Geometry check sheet. Reference: the model listing, model coordinates, mm. Face numbers are marked on the shaded views. A direction names the side the tool comes from. Give positions to 0.01 mm unless a question says otherwise; leave off trailing zeros. Loops run counter-clockwise (first coordinate to the right, second up) from the corner with the lowest first, then second, coordinate; pieces in that order, holes last.
```python
from build123d import *

# Parameters (mm, degrees)
BOSS_EXTRUDE1_DEPTH      = 50
BOSS_EXTRUDE1_DEPTH_BACK = 50
SKETCH2_R                = 50
CUT_EXTRUDE2_DEPTH       = 15
BOSS_EXTRUDE2_DEPTH      = 25
BOSS_EXTRUDE2_DEPTH_BACK = 25
SKETCH5_W                = 104.607091917
SKETCH5_H                = 30
CUT_EXTRUDE3_DEPTH       = 25
SKETCH6_W                = 40
SKETCH6_H                = 15
CUT_EXTRUDE4_DEPTH       = 81
SKETCH7_R                = 10
CUT_EXTRUDE5_DEPTH       = 61


with BuildPart() as part:
    # Sketch1 → Boss-Extrude1 (new body, two sides)
    with BuildSketch(Plane.XY) as boss_extrude1_sk:
        Polygon((0, 0), (0, 80), (30, 80), (150, 20), (150, 0), align=None)
    extrude(amount=BOSS_EXTRUDE1_DEPTH)
    extrude(boss_extrude1_sk.sketch, amount=-BOSS_EXTRUDE1_DEPTH_BACK)

    # Sketch2 → Cut-Extrude2 (cut)
    with BuildSketch(Plane.XY.offset(50)):
        Circle(SKETCH2_R)
    extrude(amount=-CUT_EXTRUDE2_DEPTH, mode=Mode.SUBTRACT)

    # Sketch4 → Boss-Extrude2 (add, two sides)
    with BuildSketch(Plane.XY) as boss_extrude2_sk:
        Polygon((70, 60), (130, 60), (130, 30), align=None)
    extrude(amount=BOSS_EXTRUDE2_DEPTH)
    extrude(boss_extrude2_sk.sketch, amount=-BOSS_EXTRUDE2_DEPTH_BACK)

    # Sketch5 → Cut-Extrude3 (cut)
    with BuildSketch(Plane(origin=(0, 60, 0), x_dir=(1, 0, 0), z_dir=(0, 1, 0))):
        with Locations((29.093290598, 0)):
            Rectangle(SKETCH5_W, SKETCH5_H)
    extrude(amount=CUT_EXTRUDE3_DEPTH, mode=Mode.SUBTRACT)

    # Sketch6 → Cut-Extrude4 (cut, through all)
    with BuildSketch(Plane.XZ):
        with Locations((100, 42.5)):
            Rectangle(SKETCH6_W, SKETCH6_H)
    extrude(amount=-CUT_EXTRUDE4_DEPTH, mode=Mode.SUBTRACT)

    # Sketch7 → Cut-Extrude5 (cut, through all)
    with BuildSketch(Plane(origin=(0, 60, 0), x_dir=(1, 0, 0), z_dir=(0, 1, 0))):
        with Locations((100, 0)):
            Circle(SKETCH7_R)
    extrude(amount=-CUT_EXTRUDE5_DEPTH, mode=Mode.SUBTRACT)


solid = part.part
```
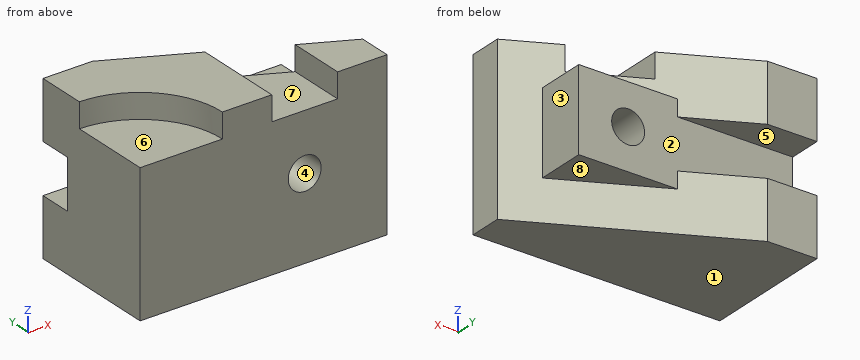
1) Sectioned sample at A-A on y = 67.5. Enter the section's corners in (x, z), plus the area to 3 significant figures.
2) Mould release check, pull along Z, two halves, no side actions. Record for the marked faces 1, 2, 3 and 4: +Z half, -Z half, draft (parallel to the pull), parting line (faces both ways), or undercut.
3) Sectioned sample at B-B on x = 100. Enter the section's corners in (y, z), plus the area to 4 significant figures.
4) Scan lines: line 1 along Z through (x, y) = (100, 43.5); line 2 along X through (y, z) = (41, 0); line 3 along X through (y, z) = (65, -30.5). Record each from-to range of solid material in increasing order.
5) Sectioned sample at D-D on z = 0. Enter the section's corners in (x, y).
6) Depth check by flat-ended pin: P1, Ø16.5, axis at y = 10.5, z = 43.5, coming from the -X side; P2, Ø2, axis at x = 112.5, z = 37.5, coming from the +Y side; P3, Ø24, axis at y = 41.5, z = 3, coming from the +X side; P4, Ø15, axis at x = 99.5, y = 40.5, coming from the +Z side. Enter the tip coordinate at first touch or a pass-through.
7) Sectioned sample at C-C on z = 44.5. Enter the section's corners in (x, y).
8) Tool access check on the marked faces 5, 6, 7 and 8. Record the directions out of +Z, -Z, +X, -X, +Y, -Y that give a thin tool (end or side, any length) a straight path to the whole face; none if there is none.
Determined:
1. outline: (0, -50) - (55, -50) - (55, -15) - (0, -15) - close; (0, 15) - (55, 15) - (55, 50) - (0, 50) - close
1. area: 3,850 mm2
2. face 1: -Z half
2. face 2: undercut
2. face 3: draft
2. face 4: undercut
3. outline: (0, -50) - (45, -50) - (45, -25) - (60, -25) - (60, -10) - (0, -10) - close; (0, 10) - (60, 10) - (60, 25) - (45, 25) - (45, 35) - (0, 35) - close
3. area: 3,375 mm2
4. line 1: z = -50 to -10, 10 to 35
4. line 2: x = 0 to 90, 110 to 130
4. line 3: x = 0 to 60
5. outline: (0, 0) - (90, 0) - (90, 60) - (0, 60) - close; (110, 0) - (150, 0) - (150, 20) - (130, 30) - (130, 60) - (110, 60) - close
6. P1: stops at x = 46.35
6. P2: passes through
6. P3: stops at x = 131
6. P4: stops at z = 35
7. outline: (0, 50) arc R50 cw to (50, 0) - (80, 0) - (80, 55) - (30, 80) - (0, 80) - close; (120, 0) - (150, 0) - (150, 20) - (120, 35) - close
8. face 5: +X, -X, +Y
8. face 6: +Z, -X, -Y
8. face 7: +Z, +Y, -Y
8. face 8: -Z, +X, +Y
